Input: part model. Units: mm. Frame: model coordinates. A direction names the side the tool comes from. Give positions to 0.01 mm unless a question says otherwise; leave off trailing zeros. Loops run counter-clockwise (first coordinate to the right, second up) from the corner with the lowest first, then second, coordinate; pieces in that order, holes last.
from build123d import *

# Parameters (mm, degrees)
EXTRU_MINCE1_DEPTH              = 28
ESQUISSE2_R                     = 2.1
ENL_V_MAT_EXTRU_1_DEPTH         = 74.86474125
R_P_TITION_LIN_AIRE1_COUNT      = 3
R_P_TITION_LIN_AIRE1_PITCH      = 8
R_P_TITION_LIN_AIRE1_COUNT_DIR2 = 7
R_P_TITION_LIN_AIRE1_PITCH_DIR2 = 8
ESQUISSE3_R                     = 2.1
ENL_V_MAT_EXTRU_2_DEPTH         = 74.86474125
R_P_TITION_LIN_AIRE2_COUNT      = 2
R_P_TITION_LIN_AIRE2_PITCH      = 8
R_P_TITION_LIN_AIRE2_COUNT_DIR2 = 7
R_P_TITION_LIN_AIRE2_PITCH_DIR2 = 8
ESQUISSE4_R                     = 11
ENL_V_MAT_EXTRU_3_DEPTH         = 74.86474125
ESQUISSE5_R                     = 1.6
ENL_V_MAT_EXTRU_4_DEPTH         = 74.86474125
R_P_TITION_CIRCULAIRE1_COUNT    = 4


with BuildPart() as part:
    # Esquisse1 → Extru.-Mince1 (new, symmetric)
    with BuildSketch(Plane.XY):
        Polygon((0, 64), (0, 0), (24, 0), (24, -3), (-3, -3), (-3, 64), align=None)
    extrude(amount=EXTRU_MINCE1_DEPTH, both=True)

    # Esquisse2 → Enlèv. mat.-Extru.1 (cut, through all)
    with BuildSketch(Plane(origin=(0, 0, 0), x_dir=(1, 0, 0), z_dir=(0, 1, 0))):
        with Locations(Location((4, -24, 0), (0, 0, 270))):
            Circle(ESQUISSE2_R)
    enl_v_mat_extru_1 = extrude(amount=-ENL_V_MAT_EXTRU_1_DEPTH, mode=Mode.SUBTRACT)

    # Répétition linéaire1: Enl_v. mat.-Extru.1 3 × 7
    with Locations(*[(i * R_P_TITION_LIN_AIRE1_PITCH, 0, -j * R_P_TITION_LIN_AIRE1_PITCH_DIR2) for i in range(R_P_TITION_LIN_AIRE1_COUNT) for j in range(R_P_TITION_LIN_AIRE1_COUNT_DIR2) if (i, j) != (0, 0)]):
        add(enl_v_mat_extru_1, mode=Mode.SUBTRACT)

    # Esquisse3 → Enlèv. mat.-Extru.2 (cut, through all)
    with BuildSketch(Plane(origin=(0, 0, 0), x_dir=(0, 0, -1), z_dir=(1, 0, 0))):
        with Locations(Location((-24, 4, 0), (0, 0, 90))):
            Circle(ESQUISSE3_R)
    enl_v_mat_extru_2 = extrude(amount=-ENL_V_MAT_EXTRU_2_DEPTH, mode=Mode.SUBTRACT)

    # Répétition linéaire2: Enl_v. mat.-Extru.2 2 × 7
    with Locations(*[(0, i * R_P_TITION_LIN_AIRE2_PITCH, -j * R_P_TITION_LIN_AIRE2_PITCH_DIR2) for i in range(R_P_TITION_LIN_AIRE2_COUNT) for j in range(R_P_TITION_LIN_AIRE2_COUNT_DIR2) if (i, j) != (0, 0)]):
        add(enl_v_mat_extru_2, mode=Mode.SUBTRACT)

    # Esquisse4 → Enlèv. mat.-Extru.3 (cut, through all)
    with BuildSketch(Plane(origin=(0, 0, 0), x_dir=(0, 0, -1), z_dir=(1, 0, 0))):
        with Locations(Location((0, 37.5, 0), (0, 0, 90))):
            Circle(ESQUISSE4_R)
    extrude(amount=-ENL_V_MAT_EXTRU_3_DEPTH, mode=Mode.SUBTRACT)

    # Esquisse5 → Enlèv. mat.-Extru.4 (cut, through all)
    with BuildSketch(Plane(origin=(0, 0, 0), x_dir=(0, 0, -1), z_dir=(1, 0, 0))):
        with Locations(Location((-15.556349186, 53.056349186, 0), (0, 0, 90))):
            Circle(ESQUISSE5_R)
    enl_v_mat_extru_4 = extrude(amount=-ENL_V_MAT_EXTRU_4_DEPTH, mode=Mode.SUBTRACT)

    # Répétition circulaire1: Enlèv. mat.-Extru.4 ×4 about axis
    r_p_tition_circulaire1_axis = Axis((0, 37.5, 0), (1, 0, 0))
    for i in range(1, R_P_TITION_CIRCULAIRE1_COUNT):
        add(enl_v_mat_extru_4.rotate(r_p_tition_circulaire1_axis, i * 360 / R_P_TITION_CIRCULAIRE1_COUNT), mode=Mode.SUBTRACT)


solid = part.part
(1) Cut plane A-A (y = 37.5). Return the cut outline in (x, z), and give its area (3 significant figures).
Values follow:
outline: (-3, -28) - (0, -28) - (0, -11) - (-3, -11) - close; (-3, 11) - (0, 11) - (0, 28) - (-3, 28) - close
area: 102 mm2
(2) Reachability of faces 1 (the cylindrical face through (3.2, -1.48, -22.06)), 2 (the flat face through (0, 25, 0)) from +Z, -Z, +X, -X, +Y, -Y: full face, straight path, thin tool, end or side. Return the list, or none.
Values follow:
face 1: +Y, -Y
face 2: +Z, -Z, +X, +Y
(3) Cut plane B-B (z = 24). Return the cut outline in (x, y).
Values follow:
outline: (-3, -3) - (1.9, -3) - (1.9, 0) - (0, 0) - (0, 1.9) - (-3, 1.9) - close; (-3, 6.1) - (0, 6.1) - (0, 9.9) - (-3, 9.9) - close; (-3, 14.1) - (0, 14.1) - (0, 64) - (-3, 64) - close; (6.1, -3) - (9.9, -3) - (9.9, 0) - (6.1, 0) - close; (14.1, -3) - (17.9, -3) - (17.9, 0) - (14.1, 0) - close; (22.1, -3) - (24, -3) - (24, 0) - (22.1, 0) - close
(4) Cut plane C-C (x = 12). Count the separate pieces of the cut face and the enclosed holes in it, and give its area (3 significant figures).
Values follow:
separate pieces: 8
enclosed holes: 0
area: 79.8 mm2
(5) Mould query, pull axis Z, two halves, no side actions, for faces 3 (the cylindrical face through (22.082, -1.479, -24.273)), 4 (the flat face through (-0.4, 20.7, 28)), 5 (the cylindrical face through (-1.479, 47.661, -4.213)), 6 (the flat face through (24, -1, 0)). Classes: +Z half, -Z half, draft (parallel to the pull), parting line (faces both ways), or undercut.
Values follow:
face 3: undercut
face 4: +Z half
face 5: undercut
face 6: draft
(6) Pin query (flat end, axial travel): pin 1 Ø4 at (y, z) = (29, 9.5) entering from +X; pin 2 Ø5 at (x, z) = (20, 8) entering from +Y. Return the tip coordinate at first contact, or that it passes through.
Values follow:
pin 1: stops at x = 0
pin 2: stops at y = 0
(7) Ray query, probe 1 along X at (y, z) = (-2, 0); probe 2 along Z at (x, y) = (-1.2, 37.5); probe 3 along Y at (x, z) = (3, -21.5). Return the intervals inside material, ascending.
Values follow:
probe 1: x = -3 to 1.9, 6.1 to 9.9, 14.1 to 17.9, 22.1 to 24
probe 2: z = -28 to -11, 11 to 28
probe 3: y = -3 to 0
